```python
from build123d import *

# Parameters (mm, degrees)
F1_DEPTH = 20


with BuildPart() as f1:
    # F0 (on Front) → F1 (new body)
    with BuildSketch(Plane.XZ):
        with BuildLine():
            ThreePointArc((-21.6, 4.8), (-24, 4), (-26.4, 4.8))
            ThreePointArc((-26.4, 4.8), (-29.826577, 5.997493), (-33.316625, 5))
            ThreePointArc((-33.316625, 5), (-34.901199, 4.255437), (-36.63325, 4))
            Line((-36.63325, 4), (-45, 4))
            Line((-45, 4), (-45, 2))
            Line((-45, 2), (-36.63325, 2))
            ThreePointArc((-36.63325, 2), (-34.323849, 2.340583), (-32.211083, 3.333333))
            ThreePointArc((-32.211083, 3.333333), (-29.884385, 3.998329), (-27.6, 3.2))
            ThreePointArc((-27.6, 3.2), (-24, 2), (-20.4, 3.2))
            ThreePointArc((-20.4, 3.2), (-18.115615, 3.998329), (-15.788917, 3.333333))
            ThreePointArc((-15.788917, 3.333333), (-13.676151, 2.340583), (-11.36675, 2))
            Line((-11.36675, 2), (-4, 2))
            Line((-4, 2), (-4, 0))
            Line((-4, 0), (0, 0))
            Line((0, 0), (0, 4))
            Line((0, 4), (-11.36675, 4))
            ThreePointArc((-11.36675, 4), (-13.098801, 4.255437), (-14.683375, 5))
            ThreePointArc((-14.683375, 5), (-18.173423, 5.997493), (-21.6, 4.8))
        make_face()
    extrude(amount=-F1_DEPTH)


solid = f1.part
```
CAD build for the part. Positions are in the model's coordinates, mm. A direction names the side the tool comes from. Coordinates: 2 decimals unless noted, no trailing zeros. Order: outer loops, then holes, each group sorted by start corner. A loop starts at its lowest first (then second) coordinate and runs counter-clockwise, first axis right, second up. Notation, with made-up numbers: M 27,46.25 L 48,46.25 A22 cw 48,63.25 Z; hole C 2,23.25 d1. An arc over 180 degrees is marked long. Write each question's results on one line, items separated by ' | '. Start each with the question number.
Q1. Cut at B-B (z = 4.4). List the corners of the cut face in (x, y), then the cut area to 3 significant figures.
Q2. Flat gauge pins, fed straight in: P1, Ø6, axis at x = -7.5, y = 13, coming from the -Z side; P2, Ø1, axis at x = -11, y = 11, coming from the +Z side; P3, Ø0.6, axis at y = 6, z = 1, coming from the -X side; P4, Ø2, axis at x = -17.5, z = 2.5, coming from the -Y side. Where does each tip first touch, or does it go through?
Q3. Cut at D-D (x = -8). List the corners of the cut face in (y, z), then the cut area to 3 significant figures.
Q4. Drill centre lines: probe 1 along X at (y, z) = (2.5, 3.1); probe 2 along X at (y, z) = (16.75, 1.95); probe 3 along X at (y, z) = (17.25, 2.7). Where is each one in solid material? Low to high. Write a range as from..to.
Q5. Which spindle directions (+Z, -Z, +X, -X, +Y, -Y) get a long thin tool onto all of the face, cutting with end or side? Do faces 1 (the flat face through (-4, 10, 1)), 2 (the flat face through (-41, 10, 4)), 3 (the flat face through (-6, 10, 4)), 4 (the cylindrical face through (-34.36, 9.86, 2.33)). Say none if no direction does.
Q6. Cut at A-A (y = 10). List the corners of the cut face in (x, z).
Q7. Cut at C-C (z = 0.6). List the corners of the cut face in (x, y), then the cut area to 3 significant figures.
Found:
1) outline: M -34.48,0 L -25.74,0 L -25.74,20 L -34.48,20 Z; M -22.26,0 L -13.52,0 L -13.52,20 L -22.26,20 Z | area: 349 mm²
2) P1: z = 2 | P2: z = 4 | P3: x = -4 | P4: through
3) outline: M 0,2 L 20,2 L 20,4 L 0,4 Z | area: 40.0 mm²
4) probe 1: -45..-32.58, -27.46..-20.54, -15.42..0 | probe 2: -4..0 | probe 3: -45..-33.36, -26.81..-21.19, -14.64..0
5) face 1: -Z, -X, +Y, -Y | face 2: +Z, -X, +Y, -Y | face 3: +Z, +X, +Y, -Y | face 4: -Z, +Y, -Y
6) outline: M -45,2 L -36.63,2 A8 ccw -32.21,3.33 A4 cw -27.6,3.2 A6 ccw -20.4,3.2 A4 cw -15.79,3.33 A8 ccw -11.37,2 L -4,2 L -4,0 L 0,0 L 0,4 L -11.37,4 A6 cw -14.68,5 A6 ccw -21.6,4.8 A4 cw -26.4,4.8 A6 ccw -33.32,5 A6 cw -36.63,4 L -45,4 Z
7) outline: M -4,0 L 0,0 L 0,20 L -4,20 Z | area: 80.0 mm²
